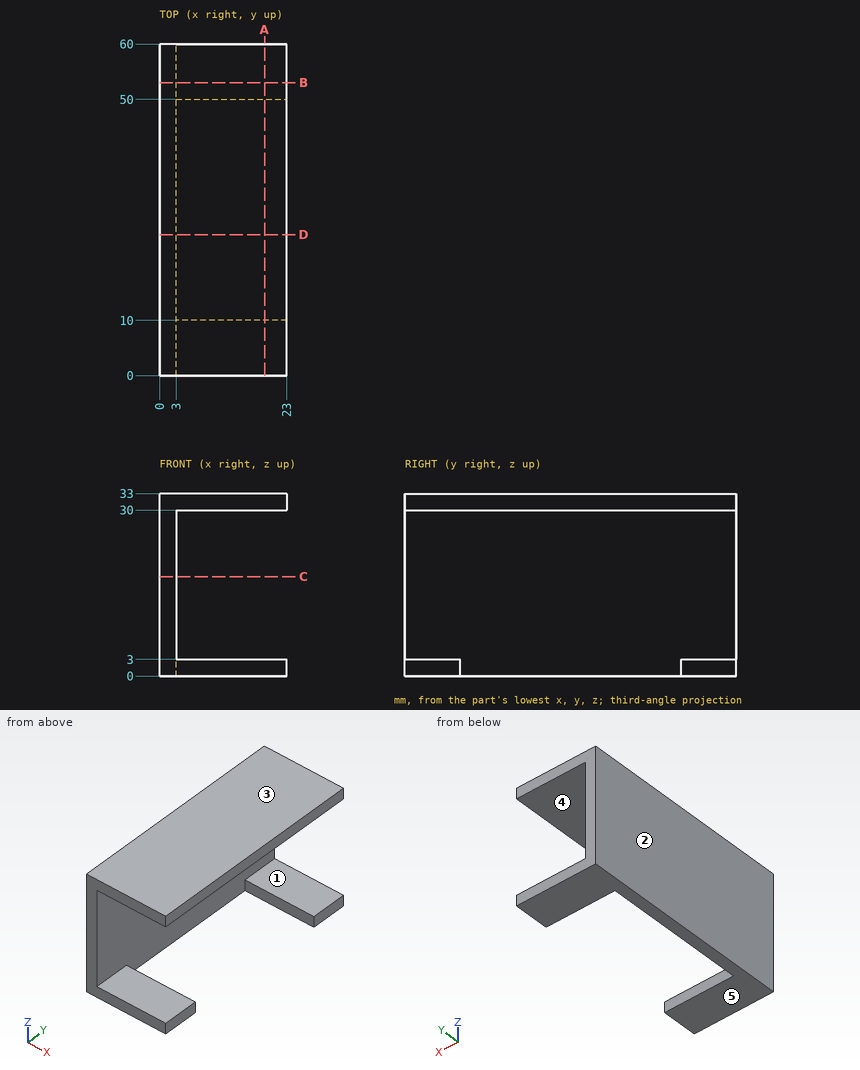
Print and shaded views of the part. All mm, measured from the part's lowest x, y and z. A direction names the side the tool comes from. Coordinates: 2 decimals unless noted, no trailing zeros. Loops run counter-clockwise (first coordinate to the right, second up) from the corner with the lowest first, then second, coordinate; pieces in that order, holes last. Notation, with made-up numbers: (82.25, 78) - (106.25, 78) arc R22 ccw to (106.25, 86) - close; hole circle Ø4 at (-40, 28.5). An arc over 180 degrees is marked (long way). Use one line per item in the form item = value. Start each with the question number.
1) Two-plate mould, pull along Z, no slides. Class the marked faces 3, 4 and 5: +Z half, -Z half, draft (parallel to the pull), parting line (faces both ways), or undercut.
2) Band-saw the part on A-A (x = 19). Give the cut face in (y, z), and give its area (3 significant figures).
3) Tool access for the marked faces 1 and 2: list every direction of +Z, -Z, +X, -X, +Y, -Y with a clear straight run to the whole face (end or side of a thin tool).
4) Band-saw the part on D-D (y = 25.5). Give the cut face in (x, z).
5) Band-saw the part on C-C (z = 18). Give the cut face in (x, y), and give its area (3 significant figures).
6) Drill centre lines: L1, parallel to X at y = 22.5, z = 27; L2, parallel to Z at x = 11, y = 41. Where is each one in solid material? Low to high. Write a range as from..to.
7) Flat gauge pins, fed straight in: pin 1 (6 mm diameter, centred on y = 49, z = 23.5, fed in from +X); pin 2 (4 mm diameter, centred on x = 6, y = 27.5, fed in from -Z); pin 3 (8 mm diameter, centred on y = 6, z = 25, fed in from -X). Where does each tip first touch, or does it go through?
8) Band-saw the part on B-B (y = 53). Give the cut face in (x, z), and give its area (3 significant figures).
Check values:
q1.face_3 = +Z half
q1.face_4 = undercut
q1.face_5 = -Z half
q2.outline = (0, 0) - (10, 0) - (10, 3) - (0, 3) - close; (0, 30) - (60, 30) - (60, 33) - (0, 33) - close; (50, 0) - (60, 0) - (60, 3) - (50, 3) - close
q2.area = 240 mm2
q3.face_1 = +X, +Y, -Y
q3.face_2 = +Z, -Z, -X, +Y, -Y
q4.outline = (0, 0) - (3, 0) - (3, 30) - (23, 30) - (23, 33) - (0, 33) - close
q5.outline = (0, 0) - (3, 0) - (3, 60) - (0, 60) - close
q5.area = 180 mm2
q6.L1 = 0..3
q6.L2 = 30..33
q7.pin_1 = 3
q7.pin_2 = 30
q7.pin_3 = 0
q8.outline = (0, 0) - (23, 0) - (23, 3) - (3, 3) - (3, 30) - (23, 30) - (23, 33) - (0, 33) - close
q8.area = 219 mm2
